```python
from build123d import *

# Parameters (mm, degrees)
EXTRUDE_THIN1_DEPTH      = 10
EXTRUDE_THIN1_DEPTH_BACK = 3


with BuildPart() as part:
    # Sketch2 → Extrude-Thin1 (new, two sides: drawn at the far end of the back side and taken through both)
    with BuildSketch(Plane.XY.offset(-EXTRUDE_THIN1_DEPTH_BACK)):
        with BuildLine():
            Line((-240.84576429, 51.220485395), (2.128944074, 13.83718169))
            ThreePointArc((2.128944074, 13.83718169), (13.841987462, 2.097470641), (6.132730824, -12.585293506))
            Line((6.132730824, -12.585293506), (-50.115721031, -39.994794473))
            ThreePointArc((-50.115721031, -39.994794473), (-53.998383655, -44.115390019), (-54.18122983, -49.77409517))
            Line((-54.18122983, -49.77409517), (-32.366451516, -113.589833173))
            ThreePointArc((-32.366451516, -113.589833173), (-34.222214173, -126.256574565), (-45.603348876, -132.11831197))
            Line((-45.603348876, -132.11831197), (-136.596329555, -132.186386844))
            ThreePointArc((-136.596329554, -132.186386844), (-136.601566486, -132.186389782), (-136.606803418, -132.186390762))
            Line((-136.606803418, -132.186390762), (-226.602303418, -132.186390762))
            ThreePointArc((-226.602303418, -132.186390762), (-233.783844459, -130.204105531), (-238.931690823, -124.818600515))
            Line((-238.931690823, -124.818600515), (-293.515400395, -23.346583433))
            ThreePointArc((-293.515400395, -23.346583433), (-290.257598601, 30.23714982), (-240.84576429, 51.220485395))
        make_face()
        with BuildLine():
            Line((-241.301966592, 48.255375033), (1.672741773, 10.872071328))
            ThreePointArc((1.672741773, 10.872071328), (10.875847292, 1.648012647), (4.818574219, -9.888444898))
            Line((4.818574219, -9.888444898), (-51.429877637, -37.297945864))
            ThreePointArc((-51.429877637, -37.297945864), (-56.768538744, -42.963764741), (-57.019952235, -50.744484323))
            Line((-57.019952235, -50.744484323), (-35.205173921, -114.560222326))
            ThreePointArc((-35.205173921, -114.560222326), (-36.663273152, -124.512661991), (-45.605593275, -129.11831281))
            Line((-45.605593275, -129.11831281), (-136.598573954, -129.186387684))
            ThreePointArc((-136.598573954, -129.186387684), (-136.602688686, -129.186389992), (-136.606803418, -129.186390762))
            Line((-136.606803418, -129.186390762), (-226.602303418, -129.186390762))
            ThreePointArc((-226.602303418, -129.186390762), (-232.244942807, -127.628880938), (-236.289679236, -123.397412711))
            Line((-236.289679236, -123.397412711), (-290.873388808, -21.925395629))
            ThreePointArc((-290.873388808, -21.925395629), (-287.807222413, 28.506353315), (-241.301966592, 48.255375033))
        make_face(mode=Mode.SUBTRACT)
    extrude(amount=EXTRUDE_THIN1_DEPTH + EXTRUDE_THIN1_DEPTH_BACK)


solid = part.part
```
Design review of the part built by this model. Coordinates are the model's own, in mm. A direction names the side the tool comes from. Coordinates: 2 decimals unless noted, no trailing zeros. Loops run counter-clockwise (first coordinate to the right, second up) from the corner with the lowest first, then second, coordinate; pieces in that order, holes last.
Q1. We need section B-B on x = -15.5. State the section outline as (y, z) points.
Reported:
outline: (-23.13, -3) - (-19.79, -3) - (-19.79, 10) - (-23.13, 10) - close; (13.51, -3) - (16.55, -3) - (16.55, 10) - (13.51, 10) - close
Q2. We need section C-C on y = -15.5. State the section outline as (x, z) points, and give its area (3 significant figures).
Reported:
outline: (-296.92, -3) - (-293.74, -3) - (-293.74, 10) - (-296.92, 10) - close; (-6.7, -3) - (0.15, -3) - (0.15, 10) - (-6.7, 10) - close
area: 130 mm2
Q3. The part is to be moulded in two halves that separate along Y. For faces 4 (the face through (-142, 35, 10)), 5 (the face through (-46.265, -82.206, 3.409)), 6 (the face through (-233.69, -130.26, 3.41)), say which applies: +Y half, -Y half, draft (parallel to the pull), parting line (faces both ways), or undercut.
Reported:
face 4: draft
face 5: undercut
face 6: -Y half
Q4. Tool access review of faces 1 (the face through (-43.427, -81.235, 3.409)), 2 (the face through (-121.06, 32.79, 3.41)), 3 (the face through (-263.2, -73.37, 3.41)): name each direction out of +Z, -Z, +X, -X, +Y, -Y from which nothing blocks a thin tool from reaching the whole face with its end or side.
Reported:
face 1: +Z, -Z, +X
face 2: +Z, -Z, +X, +Y
face 3: +Z, -Z
Q5. To check wall thickness, follow line 1 (X direction, y = 4.5, z = -1); line 2 (X direction, y = -46, z = 6.5); line 3 (Y direction, x = -179.5, z = 5). State the ranges of each line that lie inside material, in increasing order.
Reported:
line 1: x = -299.47 to -296.46, 10.04 to 13.26
line 2: x = -281.33 to -277.92, -57.55 to -54.52
line 3: y = -132.19 to -129.19, 38.75 to 41.78
Q6. For pin 1 (1.5 mm diameter, centred on x = -51.5, y = -55.5, fed in from +Z); pin 2 (5 mm diameter, centred on x = -112, z = 3, fed in from +Y); pin 3 (4 mm diameter, centred on x = -184.5, z = 1.5, fed in from +Y); pin 4 (6 mm diameter, centred on x = -28.5, z = 5, fed in from +Y), all flat-tipped, find the tip position at first contact; note any pin that passes through.
Reported:
pin 1: stops at z = 10
pin 2: stops at y = 31.78
pin 3: stops at y = 42.86
pin 4: stops at y = 19.01
